Autodesk Inventor part; units mm, degrees
ref_plane "Plan de construction4" through (0, 0, 10) normal (0, 0, 1) x (1, 0, 0)
ref_plane "YZ Plane" through (0, 0, 0) normal (1, 0, 0) x (0, 1, 0)
ref_plane "XZ Plane" through (0, 0, 0) normal (0, 1, 0) x (-1, 0, 0)
sketch "Esquisse1" plane through (0, 0, 0) normal (0, 0, 1) x (1, 0, 0)
  circle A0 centre (0, 0) radius 12.5
  dimension "d0" = 25
ref_plane "Plan de construction4" through (0, 0, 10) normal (0, 0, 1) x (1, 0, 0)
sketch "Esquisse2" plane through (0, 0, 10) normal (0, 0, 1) x (1, 0, 0)
  circle A0 centre (0, 0) radius 7.5
  dimension "d2" = 15
loft "Lissage1" add profiles "Esquisse1", "Esquisse2"
sketch "Esquisse3" plane through (0, 0, 10) normal (0, 0, 1) x (1, 0, 0)
  circle A0 centre (0, 0) radius 5
  dimension "d7" = 10
sketch "Esquisse4" plane through (0, 0, 0) normal (0, 0, -1) x (-1, 0, 0)
  circle A0 centre (0, 0) radius 10
  dimension "d8" = 20
extrude "Extrusion1" cut sketch "Esquisse3" against normal blind 22
loft "Lissage2" cut profiles "Esquisse4" section 2 edges at (-5, 0, 10)
properties part number "Frustrum"
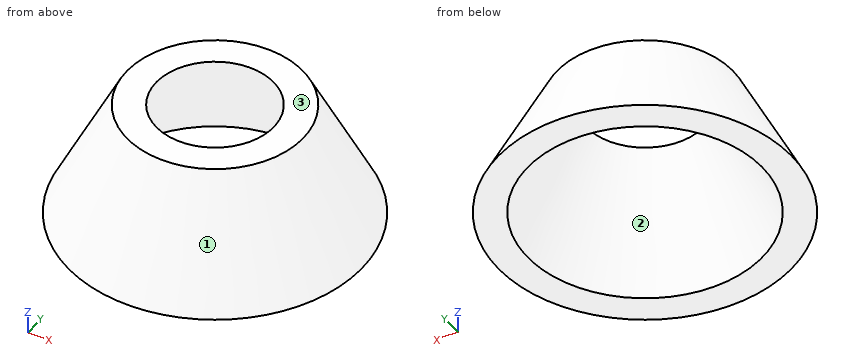
Could you check a few things on this model? Use its own coordinates, in mm. Face numbers are marked on the shaded views. Give positions to 0.01 mm unless a question says otherwise; leave off trailing zeros. Order: outer loops, then holes, each group sorted by start corner. A loop starts at its lowest first (then second) coordinate and runs counter-clockwise, first axis right, second up. Notation, with made-up numbers: (24, 25.5) - (82, 25.5) arc R26 ccw to (82, 56.5) - close; hole circle Ø3 at (47, 87.5). An arc over 180 degrees is marked (long way). One line per question, with ' | ' between items. Start each with the question number.
Item 1: I'm going to push flat-ended pins straight in: pin 1 Ø6 at (x, z) = (7.5, 6.5) entering from -Y; pin 2 Ø4 at (y, z) = (-8.5, 8.5) entering from +X; pin 3 Ø4 at (x, y) = (3.5, 2.5) entering from +Z; pin 4 Ø2 at (x, z) = (6, 5) entering from +Y. Where does each tip first touch, or does it pass through?
Item 2: I need wall thicknesses on probe 1 along Y at (x, z) = (-1.5, 5.5); probe 2 along Y at (x, z) = (1.5, 3.25); probe 3 along X at (y, z) = (-1.5, 2). Which ranges of each line are inside material? Lowest first, please. Write a range as [from, to].
Item 3: I want a section at B-B on z = 1. Write out the boundary of the cut face in (x, y), then the cut area to 3 significant figures.
Item 4: I want a section at C-C on z = 7.5. Write out the boundary of the cut face in (x, y).
Item 5: I want a section at A-A on x = 0. Write out the boundary of the cut face in (y, z), then the cut area to 3 significant figures.
Item 6: Thinking about a two-plate mould opening in Y: for the marked faces 1, 2 and 3, which applies, pulls with the +Y half, pulls with the -Y half, needs draft (parallel to the pull), parting line crosses it, or undercut?
Verdict:
1) pin 1: y = -8.8 | pin 2: x = 5.55 | pin 3: z = 10 | pin 4: y = 8.9
2) probe 1: [-9.63, -7.09], [7.09, 9.63] | probe 2: [-10.77, -8.24], [8.24, 10.77] | probe 3: [-11.4, -8.87], [8.87, 11.4]
3) outline: circle Ø24 at (0, 0); hole circle Ø19 at (0, 0) | area: 169 mm^2
4) outline: circle Ø17.5 at (0, 0); hole circle Ø12.5 at (0, 0)
5) outline: (-12.5, 0) - (-10, 0) - (-5, 10) - (-7.5, 10) - close; (5, 10) - (10, 0) - (12.5, 0) - (7.5, 10) - close | area: 50.0 mm^2
6) face 1: parting line crosses it | face 2: undercut | face 3: needs draft
